```python
from build123d import *

# Parameters (mm, degrees)
SKETCH4_R           = 2.1
BOSS_EXTRUDE3_DEPTH = 1.2
SKETCH5_W           = 84.339489928
SKETCH5_H           = 2
BOSS_EXTRUDE4_DEPTH = 2.4
SKETCH6_R           = 2.1
BOSS_EXTRUDE5_DEPTH = 1.2
SKETCH7_W           = 104.067802039
SKETCH7_H           = 60.652447956
CUT_EXTRUDE1_DEPTH  = 3.6
BOSS_EXTRUDE6_DEPTH = 1.2
CUT_EXTRUDE2_DEPTH  = 10
SKETCH10_R          = 2.1
BOSS_EXTRUDE7_DEPTH = 1.8
SKETCH11_W          = 20
SKETCH11_H          = 37
SKETCH11_H_2        = 40
SKETCH11_H_3        = 3
BOSS_EXTRUDE8_DEPTH = 2
SKETCH12_W          = 5
SKETCH12_H          = 5
CUT_EXTRUDE3_DEPTH  = 22
CHAMFER2_SIZE       = 7
FILLET1_R           = 5


with BuildPart() as part:
    # Sketch4 → Boss-Extrude3 (new body)
    with BuildSketch(Plane(origin=(0, 0, 0), x_dir=(1, 0, 0), z_dir=(0, 1, 0))):
        Polygon((39.4127274, 47.640295112), (-2.757017564, 47.640295112), (-2.757017564, 45.640295112), (39.4127274, 0.640295112), align=None)
        with Locations((22.381300815, 25.64100497)):
            Circle(SKETCH4_R, mode=Mode.SUBTRACT)
        Polygon((81.582472364, 47.640295112), (39.4127274, 47.640295112), (39.4127274, 0.640295112), (81.582472364, 45.640295112), align=None)
        with Locations((56.444153985, 25.64100497)):
            Circle(SKETCH4_R, mode=Mode.SUBTRACT)
    extrude(amount=BOSS_EXTRUDE3_DEPTH)

    # Sketch5 → Boss-Extrude4 (add)
    with BuildSketch(Plane(origin=(0, 0, 0), x_dir=(-1, 0, 0), z_dir=(0, -1, 0))):
        with Locations((-39.4127274, 46.640295112)):
            Rectangle(SKETCH5_W, SKETCH5_H)
    extrude(amount=BOSS_EXTRUDE4_DEPTH)

    # Sketch6 → Boss-Extrude5 (add)
    with BuildSketch(Plane(origin=(0, -2.4, 0), x_dir=(-1, 0, 0), z_dir=(0, -1, 0))):
        Polygon((2.757017564, 47.640295112), (-81.582472364, 47.640295112), (-81.582472364, 45.640295112), (-39.4127274, 0.640295112), (2.757017564, 45.640295112), align=None)
        with Locations((-22.381300815, 25.64100497)):
            Circle(SKETCH6_R, mode=Mode.SUBTRACT)
        with Locations((-56.444153985, 25.64100497)):
            Circle(SKETCH6_R, mode=Mode.SUBTRACT)
    extrude(amount=BOSS_EXTRUDE5_DEPTH)

    # Sketch7 → Cut-Extrude1 (cut)
    with BuildSketch(Plane(origin=(0, -3.6, 0), x_dir=(-1, 0, 0), z_dir=(0, -1, 0))):
        with Locations((-36.785683682, 25.144953811)):
            Rectangle(SKETCH7_W, SKETCH7_H)
    extrude(amount=-CUT_EXTRUDE1_DEPTH, mode=Mode.SUBTRACT)

    # Sketch8 → Boss-Extrude6 (add)
    with BuildSketch(Plane(origin=(0, 1.2, 0), x_dir=(1, 0, 0), z_dir=(0, 1, 0))):
        Polygon((-2.757017564, 47.640295112), (39.4127274, 47.640295112), (39.4127274, 62.640295112), (-30.5872726, 62.640295112), (-30.5872726, 47.640295112), align=None)
        Polygon((81.582472364, 47.640295112), (109.4127274, 47.640295112), (109.4127274, 62.640295112), (39.4127274, 62.640295112), (39.4127274, 47.640295112), align=None)
    extrude(amount=-BOSS_EXTRUDE6_DEPTH)

    # Sketch9 → Cut-Extrude2 (cut)
    with BuildSketch(Plane(origin=(0, 1.2, 0), x_dir=(1, 0, 0), z_dir=(0, 1, 0))):
        Polygon((30.041672963, 10.640295112), (48.783781837, 10.640295112), (39.4127274, 0.640295112), align=None)
    extrude(amount=-CUT_EXTRUDE2_DEPTH, mode=Mode.SUBTRACT)

    # Sketch10 → Boss-Extrude7 (add)
    with BuildSketch(Plane(origin=(0, 1.2, 0), x_dir=(1, 0, 0), z_dir=(0, 1, 0))):
        Polygon((-2.757017564, 47.640295112), (-2.757017564, 45.640295112), (30.041672963, 10.640295112), (48.783781837, 10.640295112), (81.582472364, 45.640295112), (81.582472364, 47.640295112), (109.4127274, 47.640295112), (109.4127274, 62.640295112), (-30.5872726, 62.640295112), (-30.5872726, 47.640295112), align=None)
        with Locations((22.381300815, 25.64100497)):
            Circle(SKETCH10_R, mode=Mode.SUBTRACT)
        with Locations((56.444153985, 25.64100497)):
            Circle(SKETCH10_R, mode=Mode.SUBTRACT)
    extrude(amount=BOSS_EXTRUDE7_DEPTH)

    # Sketch11 → Boss-Extrude8 (add)
    with BuildSketch(Plane(origin=(0, 0, -62.640295112), x_dir=(-1, 0, 0), z_dir=(0, 0, -1))):
        with Locations((-99.4127274, 21.5)):
            Rectangle(SKETCH11_W, SKETCH11_H)
        with Locations((-99.4127274, -20)):
            Rectangle(SKETCH11_W, SKETCH11_H_2)
        with Locations((-99.4127274, 1.5)):
            Rectangle(SKETCH11_W, SKETCH11_H_3)
        with Locations((20.5872726, 21.5)):
            Rectangle(SKETCH11_W, SKETCH11_H)
        with Locations((20.5872726, 1.5)):
            Rectangle(SKETCH11_W, SKETCH11_H_3)
        with Locations((20.5872726, -20)):
            Rectangle(SKETCH11_W, SKETCH11_H_2)
    extrude(amount=BOSS_EXTRUDE8_DEPTH)

    # Sketch12 → Cut-Extrude3 (cut)
    with BuildSketch(Plane(origin=(0, 0, -64.640295112), x_dir=(-1, 0, 0), z_dir=(0, 0, -1))):
        with Locations((-99.4127274, 25.5)):
            Rectangle(SKETCH12_W, SKETCH12_H)
        with Locations((-99.4127274, -27.5)):
            Rectangle(SKETCH12_W, SKETCH12_H)
        with Locations((20.5872726, -27.5)):
            Rectangle(SKETCH12_W, SKETCH12_H)
        with Locations((20.5872726, 25.5)):
            Rectangle(SKETCH12_W, SKETCH12_H)
    extrude(amount=-CUT_EXTRUDE3_DEPTH, mode=Mode.SUBTRACT)

    # Chamfer2
    chamfer2_edges = [part.edges().sort_by_distance(p)[0] for p in [
        (-20.5872726, 0, -62.640295112),
        (99.4127274, 3, -62.640295112),
        (99.4127274, 0, -62.640295112),
        (-20.5872726, 3, -62.640295112),
    ]]
    chamfer(chamfer2_edges, length=CHAMFER2_SIZE)

    # Fillet1
    fillet1_edges = [part.edges().sort_by_distance(p)[0] for p in [
        (109.4127274, 1.5, -47.640295112),
        (-30.5872726, 1.5, -47.640295112),
    ]]
    fillet(fillet1_edges, radius=FILLET1_R)


solid = part.part
```
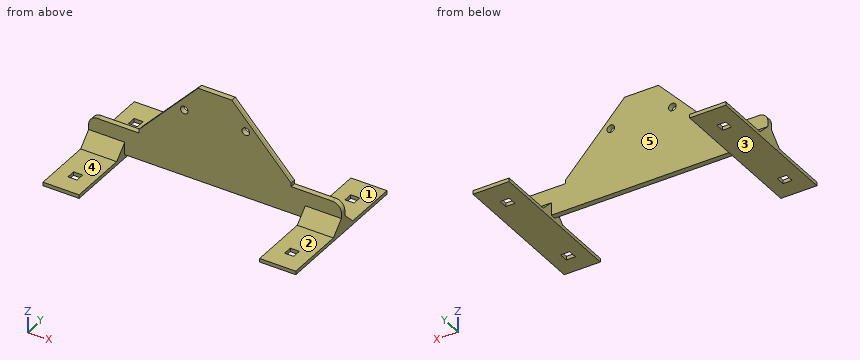
Could you check a few things on this model? Use its own coordinates, in mm. Face numbers are marked on the shaded views. A direction names the side the tool comes from. Round coordinates to 2 decimals unless told otherwise and drop trailing zeros. Write each loop counter-clockwise with the first axis right and the second up, starting at its lowest first coordinate (ties: lowest second). Pieces come first, ordered by that corner, then holes. Notation, with made-up numbers: M 5,88 L 39,88 A32 ccw 39,116 Z; hole C 78,88 d1. An arc over 180 degrees is marked long. Answer in a Markdown table with one row per item. Add a question column.
Q1. Imagine slicing it at C-C (y = 18). Please give me the cut outline in (x, z), then the cut area to 3 significant figures.
Q2. If we mould it in two halves opening along X, with no side actions, what happens to the marked faces 4 and 5? For each: +X half, -X half, draft (parallel to the pull), parting line (faces both ways), or undercut.
Q3. Imagine slicing it at A-A (x = -21). Please give me the cut outline in (y, z).
Q4. Imagine slicing it at B-B (y = -28.5). Please give me the cut outline in (x, z).
Q5. If I drill on line 1 (Y direction, x = 57, z = -35); line 2 (Z direction, x = 91, y = 10); line 3 (Z direction, x = 101, y = 6.5), over which ranges is the centre line in solid material (lowest first)? Write a range as from..to.
Q6. Will these pins go through, and if not, where does the flat tip stop? pin 1 Ø3 at (x, z) = (58, -53) entering from -Y; pin 2 Ø16 at (x, y) = (96, -27) entering from +Z; pin 3 Ø2 at (y, z) = (1.5, -46.5) entering from -X; pin 4 Ø3.5 at (x, z) = (56.44, -25.64) entering from +Y.
Q7. On a 3-axis mill with a long thin cutter (end or side, diameter ignored), from which of +Z, -Z, +X, -X, +Y, -Y can I reach the whole of each face in a straight line? I mean the marked faces 1, 2 and 3. Say none if no direction works.
Q8. Imagine slicing it at D-D (z = -17). Please give me the cut outline in (x, y).
Values:
| question | item | result |
|---|---|---|
| 1 | outline | M -30.59,-64.64 L -10.59,-64.64 L -10.59,-62.64 L -30.59,-62.64 Z; M 89.41,-64.64 L 109.41,-64.64 L 109.41,-62.64 L 89.41,-62.64 Z |
| 1 | area | 80.0 mm^2 |
| 2 | face 4 | draft |
| 2 | face 5 | undercut |
| 3 | outline | M -40,-64.64 L -30,-64.64 L -30,-62.64 L -40,-62.64 Z; M -25,-64.64 L 23,-64.64 L 23,-62.64 L 10,-62.64 L 3,-55.64 L 3,-47.64 L 0,-47.64 L 0,-55.64 L -7,-62.64 L -25,-62.64 Z; M 28,-64.64 L 40,-64.64 L 40,-62.64 L 28,-62.64 Z |
| 4 | outline | M -30.59,-64.64 L -23.09,-64.64 L -23.09,-62.64 L -30.59,-62.64 Z; M -18.09,-64.64 L -10.59,-64.64 L -10.59,-62.64 L -18.09,-62.64 Z; M 89.41,-64.64 L 96.91,-64.64 L 96.91,-62.64 L 89.41,-62.64 Z; M 101.91,-64.64 L 109.41,-64.64 L 109.41,-62.64 L 101.91,-62.64 Z |
| 5 | line 1 | 0..3 |
| 5 | line 2 | -64.64..-62.64 |
| 5 | line 3 | -64.64..-59.14 |
| 6 | pin 1 | y = 0 |
| 6 | pin 2 | z = -62.64 |
| 6 | pin 3 | x = -2.76 |
| 6 | pin 4 | through |
| 7 | face 1 | +Z, +X, -X, +Y |
| 7 | face 2 | +Z, +X, -X, -Y |
| 7 | face 3 | -Z, +X, -X, +Y, -Y |
| 8 | outline | M 24.08,0 L 54.74,0 L 54.74,3 L 24.08,3 Z |
